Can you work these out from the model? Positions are in its coordinate system, mm. A direction names the side the tool comes from. Give positions to 0.01 mm unless a question says otherwise; leave off trailing zeros. Order: outer loops, then holes, each group sorted by start corner. A loop starts at its lowest first (then second) coordinate and runs counter-clockwise, first axis right, second up.
Item 1: If I drill on line 1 along Z through (x, y) = (12.5, 0.6); line 2 along Y through (x, z) = (0.6, -20); line 3 along Y through (x, z) = (10.75, -26.5), over which ranges is the centre line in solid material (lowest first)?
Item 2: I want a section at A-A, the plane x = 12.5. Write out the boundary of the cut face in (y, z).
Item 3: If we mould it in two halves opening along Z, with no side actions, what happens to faces 1 (the flat face through (1, 14, -40)), 2 (the cylindrical face through (10.714, 0.739, -31.369)), 3 (the flat face through (1, 39, -20)), 4 (the cylindrical face through (0.739, 35.897, -18.79))? For each: +Z half, -Z half, draft (parallel to the pull), parting line (faces both ways), or undercut.
Item 4: Which directions (+Z, -Z, +X, -X, +Y, -Y) give clear straight access to the entire face, cutting with the end or side of a thin tool? Please do faces 5 (the flat face through (0, 20, -20)), 6 (the flat face through (1.5, 20, -20)).
Item 5: I want a section at C-C, the plane y = 34. Write out the boundary of the cut face in (x, z), then the cut area to 4 significant figures.
Item 6: I want a section at B-B, the plane z = -20. Write out the boundary of the cut face in (x, y).
Item 7: I want a section at D-D, the plane y = 5.5. Write out the boundary of the cut face in (x, z).
Item 8: I'm going to push flat-ended pins straight in: pin 1 Ø19 at (y, z) = (20, -19) entering from +X; pin 2 Ø12 at (x, z) = (13.5, -14) entering from +Y. Where does each tip first touch, or does it pass through?
```python
from build123d import *

# Parameters (mm, degrees)
EXTRU_MINCE1_DEPTH = 40
D_GAGEMENT_M41_D   = 4.5
D_GAGEMENT_M42_D   = 4.5


with BuildPart() as part:
    # Esquisse1 → Extru.-Mince1 (new body)
    with BuildSketch(Plane.XY):
        Polygon((0, 39), (0, 0), (25, 0), (25, 1.5), (1.5, 1.5), (1.5, 39), align=None)
    extrude(amount=-EXTRU_MINCE1_DEPTH)

    # Dégagement M41 (through all)
    with Locations(Plane(origin=(0, 1.5, 0), x_dir=(-1, 0, 0), z_dir=(0, 1, 0))):
        with Locations((-12.5, -10), (-12.5, -30)):
            Hole(D_GAGEMENT_M41_D / 2)

    # Dégagement M42 (through all)
    with Locations(Plane(origin=(1.5, 0, 0), x_dir=(0, 0, -1), z_dir=(1, 0, 0))):
        with Locations((20, 34)):
            Hole(D_GAGEMENT_M42_D / 2)


solid = part.part
```
Results list:
1. line 1: z = -40 to -32.25, -27.75 to -12.25, -7.75 to 0
1. line 2: y = 0 to 31.75, 36.25 to 39
1. line 3: y = 0 to 1.5
2. outline: (0, -40) - (1.5, -40) - (1.5, -32.25) - (0, -32.25) - close; (0, -27.75) - (1.5, -27.75) - (1.5, -12.25) - (0, -12.25) - close; (0, -7.75) - (1.5, -7.75) - (1.5, 0) - (0, 0) - close
3. face 1: -Z half
3. face 2: undercut
3. face 3: draft
3. face 4: undercut
4. face 5: +Z, -Z, -X, +Y, -Y
4. face 6: +Z, -Z, +X, +Y
5. outline: (0, -40) - (1.5, -40) - (1.5, -22.25) - (0, -22.25) - close; (0, -17.75) - (1.5, -17.75) - (1.5, 0) - (0, 0) - close
5. area: 53.25 mm2
6. outline: (0, 0) - (25, 0) - (25, 1.5) - (1.5, 1.5) - (1.5, 31.75) - (0, 31.75) - close; (0, 36.25) - (1.5, 36.25) - (1.5, 39) - (0, 39) - close
7. outline: (0, -40) - (1.5, -40) - (1.5, 0) - (0, 0) - close
8. pin 1: stops at x = 1.5
8. pin 2: stops at y = 1.5
